```python
from build123d import *

# Parameters (mm, degrees)
ESQUISSE1_W        = 20
ESQUISSE1_H        = 10.4
ESQUISSE1_R        = 1
BOSS_EXTRU_1_DEPTH = 6.4
ESQUISSE2_W        = 1
ESQUISSE2_H        = 2.5
BOSS_EXTRU_2_DEPTH = 5


with BuildPart() as part:
    # Esquisse1 → Boss.-Extru.1 (new body)
    with BuildSketch(Plane.XY):
        Rectangle(ESQUISSE1_W, ESQUISSE1_H)
        with Locations((-5, -2.2)):
            Circle(ESQUISSE1_R, mode=Mode.SUBTRACT)
        with Locations((5, -2.2)):
            Circle(ESQUISSE1_R, mode=Mode.SUBTRACT)
    extrude(amount=BOSS_EXTRU_1_DEPTH)

    # Esquisse2 → Boss.-Extru.2 (add)
    with BuildSketch(Plane.XZ.offset(5.2)):
        with Locations((-7.5, 3.2)):
            Rectangle(ESQUISSE2_W, ESQUISSE2_H)
        with Locations((0, 3.2)):
            Rectangle(ESQUISSE2_W, ESQUISSE2_H)
        with Locations((7.5, 3.2)):
            Rectangle(ESQUISSE2_W, ESQUISSE2_H)
    extrude(amount=BOSS_EXTRU_2_DEPTH)


solid = part.part
```
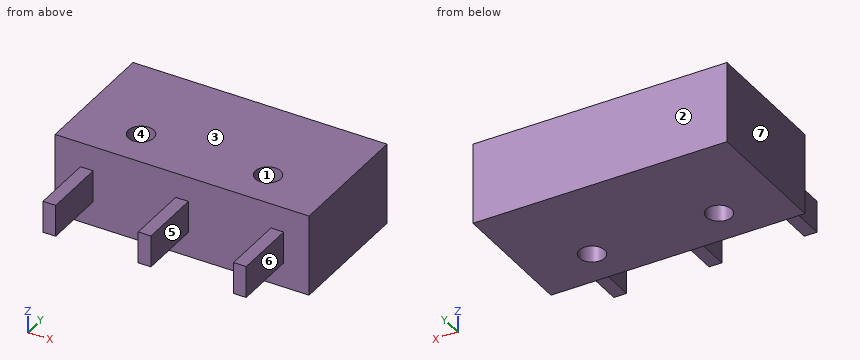
Design review of the part built by this model. Coordinates are the model's own, in mm. Face numbers are marked on the shaded views. A direction names the side the tool comes from. Give positions to 0.01 mm unless a question says otherwise; leave off trailing zeros. Loops run counter-clockwise (first coordinate to the right, second up) from the corner with the lowest first, then second, coordinate; pieces in that order, holes last. Notation, with made-up numbers: (10, 75.25) -> (54, 75.25) arc R37 ccw to (54, 111.25) -> close; hole circle Ø10 at (17.5, 20.25). An arc over 180 degrees is marked (long way). One line per item, written item: value.
Q1. We need section A-A on x = 5. Give the boundary of the cut face in (y, z).
Numbers:
outline: (-5.2, 0) -> (-3.2, 0) -> (-3.2, 6.4) -> (-5.2, 6.4) -> close; (-1.2, 0) -> (5.2, 0) -> (5.2, 6.4) -> (-1.2, 6.4) -> close
Q2. We need section C-C on z = 3.5. Give the boundary of the cut face in (x, y).
Numbers:
outline: (-10, -5.2) -> (-8, -5.2) -> (-8, -10.2) -> (-7, -10.2) -> (-7, -5.2) -> (-0.5, -5.2) -> (-0.5, -10.2) -> (0.5, -10.2) -> (0.5, -5.2) -> (7, -5.2) -> (7, -10.2) -> (8, -10.2) -> (8, -5.2) -> (10, -5.2) -> (10, 5.2) -> (-10, 5.2) -> close; hole circle Ø2 at (-5, -2.2); hole circle Ø2 at (5, -2.2)
Q3. We need section B-B on y = -2.2. Give the boundary of the cut face in (x, z), and give its area (3 significant figures).
Numbers:
outline: (-10, 0) -> (-6, 0) -> (-6, 6.4) -> (-10, 6.4) -> close; (-4, 0) -> (4, 0) -> (4, 6.4) -> (-4, 6.4) -> close; (6, 0) -> (10, 0) -> (10, 6.4) -> (6, 6.4) -> close
area: 102 mm^2
Q4. Machinability: for the marked faces 5, 6 and 7, which of the approach directions +Z, -Z, +X, -X, +Y, -Y give a long, thin tool a straight path to every point of the face, cutting with its end or side? Answer none if there is none.
Numbers:
face 5: +Z, -Z, -Y
face 6: +Z, -Z, +X, -Y
face 7: +Z, -Z, -X, +Y, -Y
Q5. For pin 1 Ø1.1 at (x, y) = (0, -7.5) entering from -Z; pin 2 Ø1.2 at (y, z) = (-6.5, 3.5) entering from +X; pin 3 Ø0.5 at (x, y) = (-7.5, -6.5) entering from +Z, all flat-tipped, find the tip position at first contact; note any pin that passes through.
Numbers:
pin 1: stops at z = 1.95
pin 2: stops at x = 8
pin 3: stops at z = 4.45
Q6. We need section D-D on y = -6. Give the boundary of the cut face in (x, z), and give its area (3 significant figures).
Numbers:
outline: (-8, 1.95) -> (-7, 1.95) -> (-7, 4.45) -> (-8, 4.45) -> close; (-0.5, 1.95) -> (0.5, 1.95) -> (0.5, 4.45) -> (-0.5, 4.45) -> close; (7, 1.95) -> (8, 1.95) -> (8, 4.45) -> (7, 4.45) -> close
area: 7.50 mm^2
Q7. Draft analysis for pull direction Y (two halves, no side actions). For the marked faces 1, 2, 3 and 4, state which applies: pulls with the +Y half, pulls with the -Y half, needs draft (parallel to the pull), parting line crosses it, or undercut.
Numbers:
face 1: undercut
face 2: pulls with the +Y half
face 3: needs draft
face 4: undercut
Q8. For L1, parallel to X at y = -8.75, z = 3.5; L2, parallel to Y at x = 5, z = 2; L3, parallel to Y at x = -2.5, z = 2.25, list the stretches that pass through material, from the lowest coordinate up.
Numbers:
L1: x = -8 to -7, -0.5 to 0.5, 7 to 8
L2: y = -5.2 to -3.2, -1.2 to 5.2
L3: y = -5.2 to 5.2
